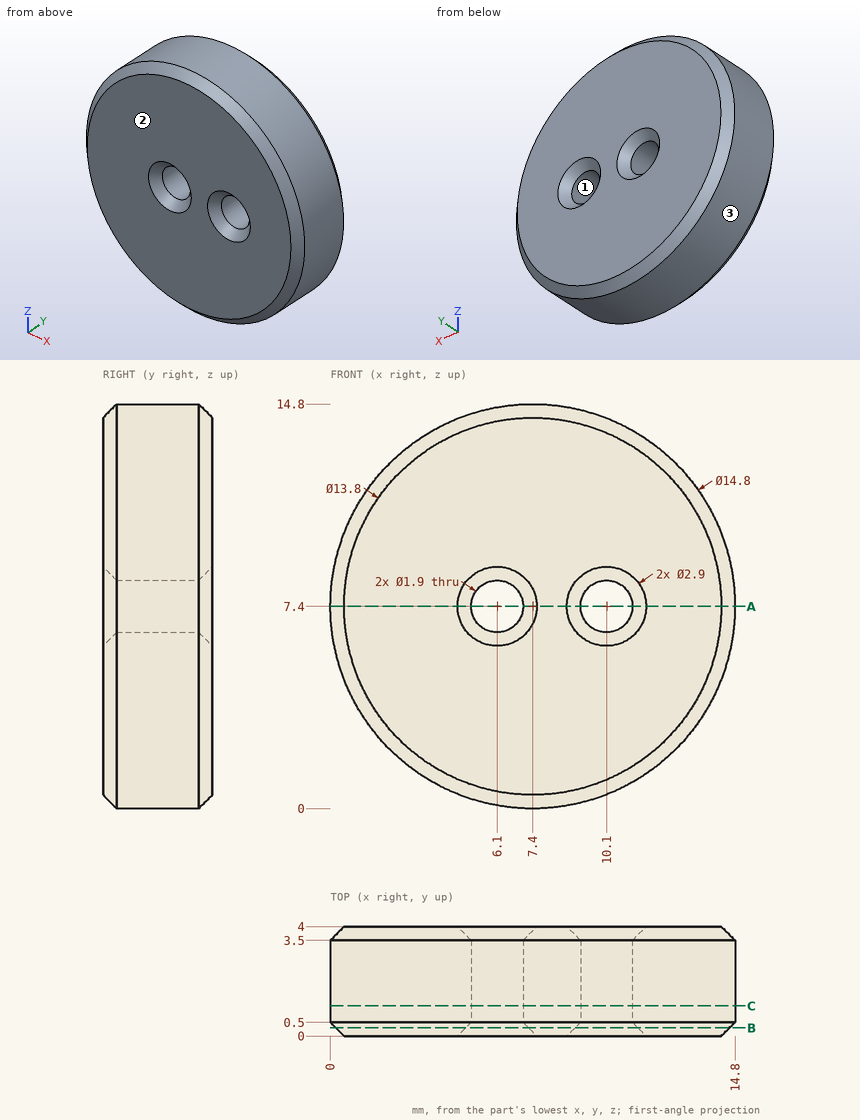
For this review, use the dimensioned drawing (mm, ordinates from the lowest corner) and the shaded views. Give positions to 0.01 mm unless a question says otherwise; leave off trailing zeros. Write each loop counter-clockwise with the first axis right and the second up, starting at its lowest first coordinate (ties: lowest second). Pieces come first, ordered by that corner, then holes. Notation, with made-up numbers: M -37.5,-3.5 L -5.5,-3.5 A32 ccw -5.5,28.5 Z; hole C 25,5 d2. An arc over 180 degrees is marked long. Answer as a JSON object with one key per item and string values. Group by question number.
Item 1: Consider section B-B on y = 0.3. Write out the cut boundary in (x, z).
Item 2: Draft analysis for pull direction Z (two halves, no side actions). For the marked faces 1, 2 and 3, state which applies: +Z half, -Z half, draft (parallel to the pull), parting line (faces both ways), or undercut.
Item 3: Consider section A-A on z = 7.4. Write out the cut boundary in (x, y).
Item 4: For probe 1 along X at (y, z) = (1.4, 7.4); probe 2 along X at (y, z) = (3.05, 6.75); probe 3 along Z at (x, y) = (9.75, 2.7), list the stretches that pass through material, from the lowest coordinate up. Write a range as [from, to].
Item 5: Consider section C-C on y = 1.1. Write out the cut boundary in (x, z), plus the area to 3 significant figures.
Item 6: For pin 1 Ø2 at (y, z) = (2.5, 13) entering from +X, flat-tipped, find the tip position at first contact; note if it passes through.
Check result:
{
 "1": {"outline": "C 7.4,7.4 d14.4; hole C 6.1,7.4 d2.3; hole C 10.1,7.4 d2.3"},
 "2": {"face 1": "undercut", "face 2": "draft", "face 3": "parting line"},
 "3": {"outline": "M 0,0.5 L 0.5,0 L 4.65,0 L 5.15,0.5 L 5.15,3.5 L 4.65,4 L 0.5,4 L 0,3.5 Z; M 7.05,0.5 L 7.55,0 L 8.65,0 L 9.15,0.5 L 9.15,3.5 L 8.65,4 L 7.55,4 L 7.05,3.5 Z; M 11.05,0.5 L 11.55,0 L 14.3,0 L 14.8,0.5 L 14.8,3.5 L 14.3,4 L 11.55,4 L 11.05,3.5 Z"},
 "4": {"probe 1": "x = [0, 5.15], [7.05, 9.15], [11.05, 14.8]", "probe 2": "x = [0.03, 5.41], [6.79, 9.41], [10.79, 14.77]", "probe 3": "z = [0.38, 6.52], [8.28, 14.42]"},
 "5": {"outline": "C 7.4,7.4 d14.8; hole C 6.1,7.4 d1.9; hole C 10.1,7.4 d1.9", "area": "166 mm^2"},
 "6": {"pin 1": "stops at x = 13.2"}
}
